Work out the finished part from the listing and answer in its coordinate system (mm). A direction names the side the tool comes from. Give positions to 0.01 mm unless a question says otherwise; leave off trailing zeros. Write each loop counter-clockwise with the first axis right and the second up, starting at its lowest first coordinate (ties: lowest second). Pieces come first, ordered by that corner, then holes. Notation, with made-up numbers: (72.5, 47.5) -> (90.5, 47.5) arc R27 ccw to (90.5, 67.5) -> close; hole circle Ø9 at (63.5, 53). An arc over 180 degrees is marked (long way). Use a Markdown table: item, result. Add a question column.
Q1. Each of these flat-tipped pins is pushed along its axis until it touches: pin 1 Ø4 at (x, y) = (16, 11) entering from -Z; pin 2 Ø4 at (y, z) = (0.5, 12.5) entering from +X; pin 3 Ø10 at (y, z) = (11.5, 7) entering from -X. Where does it stop, or does it pass through?
Q2. Section B-B, the plane y = 14 is taken. Give the vertices of the cut face in (x, z).
Q3. Section C-C, the plane x = 47 is taken. Give the vertices of the cut face in (y, z), plus the area to 3 significant figures.
Q4. Consider line 1 (Y direction, x = 32, z = 4.25); line 2 (X direction, y = 10, z = 4.75); line 3 (Z direction, x = 95, y = 12.5). Determine where each line is inside the solid, lowest interval first.
Q5. Section A-A, the plane z = 5.5 is taken. Give the vertices of the cut face in (x, y).
Q6. For a pull along Y with two mould halves and no side action, classify faces 5 (the face through (52, -3, 16)), 6 (the face through (51, 29, 16)), 7 (the face through (100.67, 13, 7)) as pulls with the +Y half, pulls with the -Y half, needs draft (parallel to the pull), parting line crosses it, or undercut.
Q7. For faces 1 (the face through (0, 13, 7)), 2 (the face through (2, 13, 7)), 3 (the face through (102.67, 13, 7)), 4 (the face through (51, 0, 7)), determine the directions among +Z, -Z, +X, -X, +Y, -Y from which every point of the face is accessible in a straight line to the end or side of a thin tool.
from build123d import *

# Parameters (mm, degrees)
SKETCH_W     = 102.67
SKETCH_H     = 25.87
SKETCH_W_2   = 98.67
SKETCH_H_2   = 21.87
PAD_DEPTH    = 15
PAD001_DEPTH = 2


with BuildPart() as part:
    # Sketch → Pad (new body)
    with BuildSketch(Plane.XY):
        with Locations((51.335, 12.935)):
            Rectangle(SKETCH_W, SKETCH_H)
        with Locations((51.335, 12.935)):
            Rectangle(SKETCH_W_2, SKETCH_H_2, mode=Mode.SUBTRACT)
    extrude(amount=PAD_DEPTH)

    # Sketch001 (on Face10 of Pad) → Pad001 (join)
    with BuildSketch(Plane.XY.offset(15)):
        with BuildLine():
            Line((0, 29), (102.648674, 29))
            ThreePointArc((105.648674, 26), (104.769994, 28.12132), (102.648674, 29))
            Line((105.648674, 26), (105.648674, 0))
            ThreePointArc((102.648674, -3), (104.769994, -2.12132), (105.648674, 0))
            Line((102.648674, -3), (0, -3))
            ThreePointArc((-3, 0), (-2.12132, -2.12132), (0, -3))
            Line((-3, 0), (-3, 26))
            ThreePointArc((0, 29), (-2.12132, 28.12132), (-3, 26))
        make_face()
    extrude(amount=PAD001_DEPTH)


solid = part.part
Result set:
| question | item | result |
|---|---|---|
| 1 | pin 1 | stops at z = 15 |
| 1 | pin 2 | stops at x = 102.67 |
| 1 | pin 3 | stops at x = 0 |
| 2 | outline | (-3, 15) -> (0, 15) -> (0, 0) -> (2, 0) -> (2, 15) -> (100.67, 15) -> (100.67, 0) -> (102.67, 0) -> (102.67, 15) -> (105.65, 15) -> (105.65, 17) -> (-3, 17) -> close |
| 3 | outline | (-3, 15) -> (0, 15) -> (0, 0) -> (2, 0) -> (2, 15) -> (23.87, 15) -> (23.87, 0) -> (25.87, 0) -> (25.87, 15) -> (29, 15) -> (29, 17) -> (-3, 17) -> close |
| 3 | area | 124 mm2 |
| 4 | line 1 | y = 0 to 2, 23.87 to 25.87 |
| 4 | line 2 | x = 0 to 2, 100.67 to 102.67 |
| 4 | line 3 | z = 15 to 17 |
| 5 | outline | (0, 0) -> (102.67, 0) -> (102.67, 25.87) -> (0, 25.87) -> close; hole (2, 2) -> (100.67, 2) -> (100.67, 23.87) -> (2, 23.87) -> close |
| 6 | face 5 | pulls with the -Y half |
| 6 | face 6 | pulls with the +Y half |
| 6 | face 7 | undercut |
| 7 | face 1 | -Z, -X, +Y, -Y |
| 7 | face 2 | -Z |
| 7 | face 3 | -Z, +X, +Y, -Y |
| 7 | face 4 | -Z, +X, -X, -Y |
